Work out the finished part from the listing and answer in its coordinate system (mm). A direction names the side the tool comes from. Coordinates: 2 decimals unless noted, no trailing zeros. Order: outer loops, then holes, each group sorted by start corner. A loop starts at its lowest first (then second) coordinate and runs counter-clockwise, first axis right, second up. Notation, with made-up numbers: (60, -4) -> (99, -4) arc R37 cw to (99, 32) -> close; hole circle Ø6 at (65, -24). An arc over 180 degrees is marked (long way). Answer as CSV lines item,"result". Start each with the question number.
Item 1: Straight lines are drawn through the part: L1, parallel to X at y = 6, z = 4.25; L2, parallel to Y at x = -6, z = 3; L3, parallel to Y at x = -7, z = 1. For each, find the intervals that lie inside material, in ascending order.
Item 2: Which of the six approach directions +Z, -Z, +X, -X, +Y, -Y give full straight-line access (tool end or side, diameter ignored) to faces 4 (the face through (7.115, 10.028, 3.613)), 5 (the face through (8, 0, 3)), 6 (the face through (3.8, 12, 3)), 7 (the face through (-13.9, 6.2, 0)), 8 (the face through (3, 4, 3))?
Item 3: Section B-B (y = 6) is taken. Write down the section's boundary in (x, z), then the cut area to 3 significant figures.
Item 4: For a pull along X with two mould halves and no side action, classify faces 1 (the face through (-18.413, 18.902, 2.958)), 2 (the face through (9, 10, 3)), 3 (the face through (5.6, 0.2, 0.8)) as pulls with the +X half, pulls with the -X half, needs draft (parallel to the pull), parting line crosses it, or undercut.
Item 5: Each of these flat-tipped pins is pushed along its axis until it touches: pin 1 Ø1 at (y, z) = (9.5, 5) entering from -X; pin 2 Ø0.8 at (x, z) = (7.5, 1.5) entering from +Y; pin 3 Ø1 at (x, z) = (3.5, 5) entering from +Y; pin 4 Ø10 at (x, y) = (-9, -3) entering from -Z. Where does it stop, or does it pass through?
Item 6: Section D-D (x = -18) is taken. Write down the section's boundary in (y, z).
Item 7: Section C-C (x = -8) is taken. Write down the section's boundary in (y, z), then the cut area to 3 significant figures.
Item 8: Section A-A (z = 3.75) is taken. Write down the section's boundary in (x, y), then the cut area to 3 significant figures.
Autodesk Inventor part; units mm, degrees
ref_plane "YZ Plane" through (0, 0, 0) normal (1, 0, 0) x (0, 1, 0)
ref_plane "XZ Plane" through (0, 0, 0) normal (0, 1, 0) x (-1, 0, 0)
ref_plane "XY Plane" through (0, 0, 0) normal (0, 0, 1) x (1, 0, 0)
sketch "スケッチ1" plane through (0, 0, 0) normal (0, 0, 1) x (1, 0, 0)
  line L0 (9, 0) -> (9, 4)
  line L1 (9, 12) -> (2.2731, 12)
  line L2 (0, 8) -> (9, 8)
  line L3 (0, 4) -> (9, 4)
  line L4 (9, 8) -> (9, 12)
  arc A0 (0, 8) -> (0, 4) centre (-5.7099, 6) ccw
  line L5 (2.2731, 12) -> (0, 14.2779)
  line L6 (2.2731, 0) -> (-5.7099, -8)
  line L7 (-5.7099, 20) -> (-15.7099, 20)
  line L8 (-5.7099, -8) -> (-15.7099, -8)
  line L9 (-15.7099, 20) -> (-25.7698, 20)
  line L10 (-25.7698, 20) -> (-25.7698, -8)
  line L11 (-25.7698, -8) -> (-15.7099, -8)
  line L12 (2.2731, 0) -> (9, 0)
  line L13 (0, 14.2779) -> (-5.7099, 20)
  point P0 (0, 0)
  point P1 (4.5, 12)
  point P2 (4.5, 0)
  point P3 (4.5, 4)
  point P4 (-25.7099, 6)
  dimension "d4" = 12.1
  dimension "d5" = 4
  dimension "d6" = 14
  dimension "d7" = 14
  dimension "d8" = 10
  dimension "d9" = 10
  dimension "d10" = 20
  dimension "d12" = 14
extrude "押し出し1" add sketch "スケッチ1" along normal blind 6
sketch "スケッチ2" plane through (0, 0, 6) normal (0, 0, 1) x (1, 0, 0)
  circle A0 centre (5.6365, 13.3) radius 1.5
  line L0 (9, 8) -> (9, 12)
  line L1 (11.5477, 6) -> (-28.1936, 6) construction
  line L2 (9, 12) -> (2.2731, 12)
  circle A1 centre (5.6365, -1.3) radius 1.5
  point P0 (0, 0)
  point P1 (4.8882, 12)
  point P2 (6.3849, 12)
  dimension "d15" = 3
  dimension "d16" = 3.3635
  dimension "d17" = 1.3
extrude "押し出し2" cut sketch "スケッチ2" against normal blind 6 contours A0 L2 | A1 picked at (5.4614, 13.0013)
sketch "スケッチ3" plane through (0, 0, 6) normal (0, 0, 1) x (1, 0, 0)
  circle A0 centre (5.6365, 13.3) radius 1.5
  line L0 (9, 12) -> (2.2731, 12)
  point P0 (0, 0)
  point P1 (4.8882, 12)
  point P2 (6.3849, 12)
  dimension "d20" = 3
  dimension "d21" = 1.3
extrude "押し出し3" add sketch "スケッチ3" against normal blind 6 contours A0 L0 picked at (5.4614, 13.0013)
sketch "スケッチ4" plane through (0, 0, 6) normal (0, 0, 1) x (1, 0, 0)
  arc A0 (6.3849, 12) -> (4.8882, 12) centre (5.6365, 13.3) ccw
  circle A1 centre (5.6365, 13.3) radius 1.5
  point P0 (0, 0)
  dimension "d24" = 3
extrude "押し出し4" cut sketch "スケッチ4" against normal blind 6
fillet "フィレット1" radius 5 1 edges at (-25.7698, 20, 3)
fillet "フィレット2" radius 5 1 edges at (-25.7698, -8, 3)
fillet "フィレット3" radius 3 4 edges at (-5.7099, -8, 3) (2.2731, 0, 3) (-5.7099, 20, 3) (2.2731, 12, 3)
sketch "スケッチ6" plane through (0, 4, 0) normal (0, 1, 0) x (1, 0, 0)
  point P0 (0, 0)
sketch "スケッチ7" plane through (4.8882, 12, 6) normal (0, 1, 0) x (1, 0, 0)
  circle A0 centre (0.7488, 3) radius 1.6
  line L0 (1.4967, 0) -> (0, 0)
  line L1 (4.1118, 6) -> (4.1118, 0)
  point P0 (-4.8882, 6)
  point P1 (0.7483, 0)
  dimension "d43" = 3.2
  dimension "d44" = 3
  dimension "d45" = 3.363
extrude "押し出し5" cut sketch "スケッチ7" against normal blind 28
sketch "スケッチ11" plane through (0, 0, 6) normal (0, 0, 1) x (1, 0, 0)
  line L0 (-6.9544, 20) -> (-20.7698, 20)
  line L1 (-20.7698, 20) -> (-6.9544, 20)
  arc A0 (1.394, 12.8809) -> (3.5176, 12) centre (3.5176, 15) ccw
  line L2 (0, 20) -> (1.3068, 17.0279)
  arc A1 (1.394, 12.8809) -> (3.5176, 12) centre (3.5176, 15) ccw
  arc A2 (-4.8308, 19.1191) -> (-6.9544, 20) centre (-6.9544, 17) ccw
  arc A3 (-4.8308, 19.1191) -> (-6.9544, 20) centre (-6.9544, 17) ccw
  line L3 (1.394, 12.8809) -> (-4.8308, 19.1191)
  line L4 (-4.8308, 19.1191) -> (1.394, 12.8809)
  arc A4 (0, 8) -> (0, 4) centre (-5.7099, 6) ccw
  line L5 (-11.7599, 6) -> (12.1155, 6) construction
  line L6 (-20.7698, -8) -> (0, -8)
  line L7 (0, -8) -> (3.5176, 0)
  arc A5 (-6.9544, -8) -> (-4.8308, -7.1191) centre (-6.9544, -5) ccw
  line L8 (1.394, -0.8809) -> (-4.8308, -7.1191)
  line L9 (-6.9544, 20) -> (0, 20)
  line L10 (1.3068, 17.0279) -> (3.5176, 12)
  arc A6 (3.5176, 0) -> (1.394, -0.8809) centre (3.5176, -3) ccw
  point P0 (0, 0)
extrude "押し出し6" add sketch "スケッチ11" against normal blind 6
sketch "スケッチ12" plane through (0, 0, 6) normal (0, 0, 1) x (1, 0, 0)
  arc A0 (0, 8) -> (0, 4) centre (-5.7099, 6) ccw
  point P0 (0, 0)
  point P1 (-15.7099, 6)
  point P2 (-5.7099, 16)
  point P3 (-5.7099, -4)
  dimension "d74" = 10
  dimension "d76" = 10
  dimension "d77" = 10
hole "穴4" at (-15.7099, 6, 6) at (-5.7099, 16, 6) at (-5.7099, -4, 6) direction (0, 0, -1) diameter 3.2 end through all
sketch "スケッチ13" plane through (0, 0, 6) normal (0, 0, 1) x (1, 0, 0)
  line L0 (-20.7698, -8) -> (0, -8)
  line L1 (0, 20) -> (-20.7698, 20)
  line L2 (-18.7698, 20) -> (-18.7698, -8) construction
  line L3 (-25.7698, 15) -> (-25.7698, -3)
  arc A0 (-18.7698, 20) -> (-18.7698, -8) centre (6.3784, 6) ccw
  line L4 (-18.7698, 20) -> (-29.3351, 20)
  line L5 (-29.3351, 20) -> (-29.3351, -8)
  line L6 (-29.3351, -8) -> (-18.7698, -8)
  point P0 (0, 0)
  dimension "d85" = 7
extrude "押し出し7" cut sketch "スケッチ13" against normal blind 6
fillet "フィレット4" radius 6 1 edges at (-18.7698, 20, 3)
fillet "フィレット5" radius 6 1 edges at (-18.7698, -8, 3)
properties part number "射出_腕固定" material "ポリカーボネート、クリア"
Checked values:
1,L1,"x = -22.4 to -17.31, -14.11 to -11.76"
1,L2,"y = -8 to -5.57, -2.43 to -0.04, 12.04 to 14.43, 17.57 to 20"
1,L3,"y = -8 to -4.95, -3.05 to 0.09, 11.91 to 15.05, 16.95 to 20"
2,face 4,"+Y, -Y"
2,face 5,"+Z, -Z, +X, -Y"
2,face 6,"+Z, -Z, +X, +Y"
2,face 7,"-Z, +X, -X, +Y, -Y"
2,face 8,"+Z, -Z, +X"
3,outline,"(-22.4, 0) -> (-17.31, 0) -> (-17.31, 6) -> (-22.4, 6) -> close; (-14.11, 0) -> (-11.76, 0) -> (-11.76, 6) -> (-14.11, 6) -> close"
3,area,"44.7 mm^2"
4,face 1,"pulls with the -X half"
4,face 2,"pulls with the +X half"
4,face 3,"undercut"
5,pin 1,"stops at x = -22.25"
5,pin 2,"stops at y = 12"
5,pin 3,"stops at y = 13.18"
5,pin 4,"stops at z = 0"
6,outline,"(-7.17, 0) -> (19.17, 0) -> (19.17, 6) -> (-7.17, 6) -> close"
7,outline,"(-8, 0) -> (0.4, 0) -> (0.4, 6) -> (-8, 6) -> close; (11.6, 0) -> (20, 0) -> (20, 6) -> (11.6, 6) -> close"
7,area,"101 mm^2"
8,outline,"(-20.57, -4.11) arc R6 ccw to (-14.95, -8) -> (0, -8) -> (3.52, 0) -> (4.22, 0) -> (4.22, 4) -> (0, 4) arc R6.05 cw (long way) to (0, 8) -> (4.22, 8) -> (4.22, 12) -> (3.52, 12) -> (1.31, 17.03) -> (0, 20) -> (-14.95, 20) arc R6 ccw to (-20.57, 16.11) arc R28.78 ccw to start; (7.05, 0) -> (9, 0) -> (9, 4) -> (7.05, 4) -> close; (7.05, 8) -> (9, 8) -> (9, 12) -> (7.05, 12) -> close; hole circle Ø3.2 at (-15.71, 6); hole circle Ø3.2 at (-5.71, -4); hole circle Ø3.2 at (-5.71, 16)"
8,area,"528 mm^2"
